from build123d import *

# Parameters (mm, degrees)
F0_W     = 150
F0_H     = 50
F1_DEPTH = 10
F2_W     = 100
F2_H     = 20
F3_DEPTH = 35
F5_DEPTH = 35.001
F6_W     = 15
F6_H     = 10
F7_DEPTH = 125.001


with BuildPart() as f1:
    # F0 (on Top) → F1 (new body)
    with BuildSketch(Plane.XY):
        with Locations((75, 25)):
            Rectangle(F0_W, F0_H)
    extrude(amount=F1_DEPTH)

    # F2 (on face) → F3 (join)
    with BuildSketch(Plane.XY.offset(10)):
        with Locations((75, 25)):
            Rectangle(F2_W, F2_H)
    extrude(amount=F3_DEPTH)

    # F4 (on face) → F5 (cut, through all)
    with BuildSketch(Plane.XZ.offset(-15)):
        with BuildLine():
            Line((41, 45), (34, 45))
            Line((34, 45), (34, 19.5))
            ThreePointArc((34, 19.5), (37.5, 16), (41, 19.5))
            Line((41, 19.5), (41, 45))
        make_face()
        with BuildLine():
            Line((116, 19.5), (116, 45))
            Line((116, 45), (109, 45))
            Line((109, 45), (109, 19.5))
            ThreePointArc((109, 19.5), (112.5, 16), (116, 19.5))
        make_face()
        with BuildLine():
            Line((66, 45), (59, 45))
            Line((59, 45), (59, 19.5))
            ThreePointArc((59, 19.5), (62.5, 16), (66, 19.5))
            Line((66, 19.5), (66, 45))
        make_face()
        with BuildLine():
            ThreePointArc((84, 19.5), (87.5, 16), (91, 19.5))
            Line((91, 19.5), (91, 45))
            Line((91, 45), (84, 45))
            Line((84, 45), (84, 19.5))
        make_face()
    extrude(amount=-F5_DEPTH, mode=Mode.SUBTRACT)

    # F6 (on face) → F7 (cut, through all)
    with BuildSketch(Plane.YZ.offset(125)):
        with Locations((25, 32)):
            Rectangle(F6_W, F6_H)
    extrude(amount=-F7_DEPTH, mode=Mode.SUBTRACT)


solid = f1.part
Verification items for the finished model (mm, model axes). A direction names the side the tool comes from. Coordinates: 2 decimals unless noted, no trailing zeros. Loops run counter-clockwise (first coordinate to the right, second up) from the corner with the lowest first, then second, coordinate; pieces in that order, holes last. Notation, with made-up numbers: (-33.75, -3) -> (-8.75, -3) arc R25 ccw to (-8.75, 15) -> close; hole circle Ø9 at (2, 43). An arc over 180 degrees is marked (long way). Answer as a JSON object with one key per item and string values. Group by question number.
Item 1: Sectioned sample at A-A on x = 99. Record the boundary of the cut face in (y, z).
Item 2: Depth check by flat-ended pin: pin 1 (10 mm diameter, centred on x = 31, z = 34.5, fed in from +Y); pin 2 (8 mm diameter, centred on y = 36, z = 18.5, fed in from +X); pin 3 (6 mm diameter, centred on y = 25.5, z = 27, fed in from -X). Enter the tip coordinate at first touch or a pass-through.
Item 3: Sectioned sample at C-C on y = 21.5. State how many separate pieces and enclosed holes the cut face has, plus the area to 3 significant figures.
Item 4: Scan lines: probe 1 along Y at (x, z) = (56, 35.5); probe 2 along Z at (x, y) = (47, 26); probe 3 along Z at (x, y) = (70.5, 11). Record each from-to range of solid material in increasing order.
Item 5: Mould release check, pull along Y, two halves, no side actions. Record for faces 1 (the flat face through (50, 25, 45)), 2 (the flat face through (74, 0, 5)), 3 (the flat face through (30, 32.5, 32)): +Y half, -Y half, draft (parallel to the pull), parting line (faces both ways), or undercut.
Item 6: Tool access check on faces 4 (the flat face through (91, 25, 38)), 5 (the flat face through (25, 25, 23)), 6 (the flat face through (30, 17.5, 32)), 7 (the flat face through (29, 25, 45)). Record the directions out of +Z, -Z, +X, -X, +Y, -Y that give a thin tool (end or side, any length) a straight path to the whole face; none if there is none.
Item 7: Sectioned sample at B-B on x = 37.5. Record the boundary of the cut face in (y, z).
Evaluation:
{
 "1": {"outline": "(0, 0) -> (50, 0) -> (50, 10) -> (35, 10) -> (35, 45) -> (15, 45) -> (15, 10) -> (0, 10) -> close; hole (17.5, 27) -> (32.5, 27) -> (32.5, 37) -> (17.5, 37) -> close"},
 "2": {"pin 1": "stops at y = 35", "pin 2": "stops at x = 125", "pin 3": "stops at x = 25"},
 "3": {"separate pieces": "6", "enclosed holes": "0", "area": "3,490 mm²"},
 "4": {"probe 1": "y = 15 to 17.5, 32.5 to 35", "probe 2": "z = 0 to 27, 37 to 45", "probe 3": "z = 0 to 10"},
 "5": {"face 1": "draft", "face 2": "-Y half", "face 3": "undercut"},
 "6": {"face 4": "+Z, +Y, -Y", "face 5": "+Z, -X, +Y, -Y", "face 6": "+X, -X", "face 7": "+Z, +X, -X, +Y, -Y"},
 "7": {"outline": "(0, 0) -> (50, 0) -> (50, 10) -> (35, 10) -> (35, 16) -> (15, 16) -> (15, 10) -> (0, 10) -> close"}
}
